Build history of the part. All positions in model axes, mm. Give positions to 0.01 mm unless a question says otherwise; leave off trailing zeros. Loops run counter-clockwise (first coordinate to the right, second up) from the corner with the lowest first, then second, coordinate; pieces in that order, holes last. Notation, with made-up numbers: (-20.5, 61) -> (28.5, 61) arc R19 ccw to (28.5, 92) -> close; hole circle Ø2 at (-32, 78). An arc over 180 degrees is marked (long way). Answer as a JSON object with one key per item and string values. Group by question number.
from build123d import *

# Parameters (mm, degrees)
F0_R     = 3.175
F1_DEPTH = 69.85
F2_W     = 9.525
F2_H     = 0.8128
F3_DEPTH = 12.7


with BuildPart() as f1:
    # F0 (on Right) → F1 (new body)
    with BuildSketch(Plane.YZ):
        Circle(F0_R)
    extrude(amount=F1_DEPTH)

    # F2 (on Front) → F3 (cut, symmetric)
    with BuildSketch(Plane.XZ):
        with Locations((65.0875, 2.7686)):
            Rectangle(F2_W, F2_H)
        with Locations((4.7625, 2.7686)):
            Rectangle(F2_W, F2_H)
    extrude(amount=F3_DEPTH, both=True, mode=Mode.SUBTRACT)


solid = f1.part
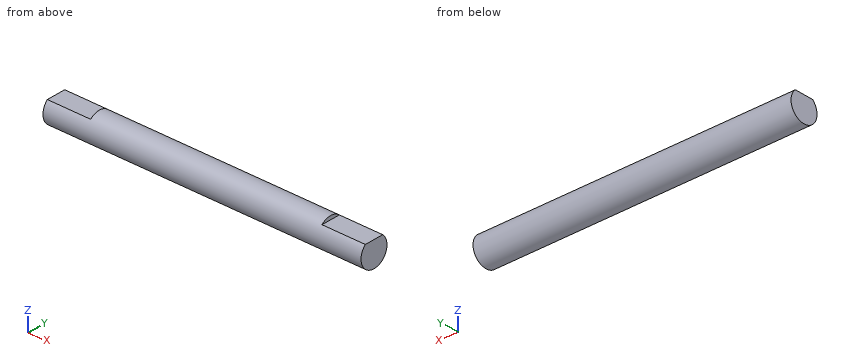
(1) Pin check, flat tips, straight feed: pin 1 (1.5 mm diameter, centred on x = 8.5, y = 0.5, fed in from +Z); pin 2 (1 mm diameter, centred on x = 23.5, y = 1.5, fed in from +Z); pin 3 (1 mm diameter, centred on x = 24.5, y = -1, fed in from +Z). Stop position of each tip, or through.
(2) Probe line 1 along Y through (x, z) = (45.5, -0.25); line 2 along Z through (x, y) = (7, 1.75); line 3 along Z through (x, y) = (15.5, 2). List the from-to ranges inside material, lowest first. Write a range as [from, to].
(3) Saw through at B-B on x = 40.5. List the corners of the cut face in (y, z) (3 decimals), plus the area to 3 significant figures.
(4) Saw through at C-C on z = 1.25. List the corners of the cut face in (x, y), plus the area to 3 significant figures.
(5) Saw through at A-A on y = 0. List the corners of the cut face in (x, z) (3 decimals), plus the area to 3 significant figures.
Calculated:
{
 "1": {"pin 1": "stops at z = 2.36", "pin 2": "stops at z = 3.01", "pin 3": "stops at z = 3.14"},
 "2": {"line 1": "y = [-3.17, 3.17]", "line 2": "z = [-2.65, 2.36]", "line 3": "z = [-2.47, 2.47]"},
 "3": {"outline": "circle Ø6.35 at (0, 0)", "area": "31.7 mm^2"},
 "4": {"outline": "(0, -2.92) -> (69.85, -2.92) -> (69.85, 2.92) -> (0, 2.92) -> close", "area": "408 mm^2"},
 "5": {"outline": "(0, -3.175) -> (69.85, -3.175) -> (69.85, 2.362) -> (60.325, 2.362) -> (60.325, 3.175) -> (9.525, 3.175) -> (9.525, 2.362) -> (0, 2.362) -> close", "area": "428 mm^2"}
}
